```python
from build123d import *

# Parameters (mm, degrees)
BOSS_EXTRUDE1_DEPTH = 6.25
SKETCH2_R           = 2
CUT_EXTRUDE1_DEPTH  = 6.35


with BuildPart() as part:
    # Sketch1 → Boss-Extrude1 (new body)
    with BuildSketch(Plane(origin=(0, 0, 0), x_dir=(1, 0, 0), z_dir=(0, 1, 0))):
        with BuildLine():
            Line((111.125, 0), (187.325, 0))
            ThreePointArc((187.325, 0), (132.458777786, -132.458777786), (0, -187.325))
            Line((0, -187.325), (0, -111.125))
            ThreePointArc((0, -111.125), (78.577241059, -78.577241059), (111.125, 0))
        make_face()
    extrude(amount=BOSS_EXTRUDE1_DEPTH)

    # Sketch2 → Cut-Extrude1 (cut)
    with BuildSketch(Plane(origin=(0, 6.25, 0), x_dir=(1, 0, 0), z_dir=(0, 1, 0))):
        with Locations(Location((21.777652082, -123.507202325, 0), (0, 0, 270))):
            Circle(SKETCH2_R)
        with Locations(Location((123.507202325, -21.777652082, 0), (0, 0, 270))):
            Circle(SKETCH2_R)
        with Locations(Location((26.739648758, -151.648083867, 0), (0, 0, 270))):
            Circle(SKETCH2_R)
        with Locations(Location((151.648083867, -26.739648758, 0), (0, 0, 270))):
            Circle(SKETCH2_R)
    extrude(amount=-CUT_EXTRUDE1_DEPTH, mode=Mode.SUBTRACT)


solid = part.part
```
Source: CAD feature listing. Evaluate the final solid. Frame: model axes, mm. Give positions to 0.01 mm unless a question says otherwise; leave off trailing zeros. Loops run counter-clockwise (first coordinate to the right, second up) from the corner with the lowest first, then second, coordinate; pieces in that order, holes last. Notation, with made-up numbers: (-21, -32) -> (0, -32) arc R16 cw to (0, -14) -> close; hole circle Ø6 at (87, 70.5). An arc over 180 degrees is marked (long way). Put each result on its own line as item: value. Start each with the question number.
1) Material intervals for probe 1 along Z at (x, y) = (25, 4.25); probe 2 along X at (y, z) = (3, 25.5); probe 3 along X at (y, z) = (2.5, 116.5), sorted ascending.
2) Draft query along Z for faces 1 (the face through (133.9, 3.1, 131)), 2 (the face through (28.43, 3.17, 152.72)), 3 (the face through (95, 6.25, 92)). Return one class per face: released by +Z, released by -Z, zero draft, split by the parting line, or undercut.
3) Contact query for flat-ended pins moving along their axis: P1, Ø1.5, axis at y = 2, z = 119.5, coming from the +X side; P2, Ø3, axis at x = 38.5, y = 5, coming from the -Z side; P3, Ø1, axis at x = 90.5, y = 2, coming from the +Z side. Output: stop coordinate, or through.
4) Cut plane C-C (x = 99.5). Return loops of the section in (y, z), then the cut area to 3 significant figures.
5) Cut plane B-B (z = 146). Return loops of the section in (x, y).
6) Cut plane A-A (y = 2). Return loops of the section in (x, z) (3 decimals), then the cut area to 3 significant figures.
Results are:
1. probe 1: z = 108.28 to 150.66, 152.63 to 185.65
1. probe 2: x = 108.16 to 150.08, 153.22 to 185.58
1. probe 3: x = 0 to 146.69
2. face 1: released by +Z
2. face 2: undercut
2. face 3: zero draft
3. P1: stops at x = 144.88
3. P2: stops at z = 103.68
3. P3: stops at z = 164.29
4. outline: (0, 49.48) -> (6.25, 49.48) -> (6.25, 158.71) -> (0, 158.71) -> close
4. area: 683 mm2
5. outline: (0, 0) -> (117.37, 0) -> (117.37, 6.25) -> (0, 6.25) -> close
6. outline: (0, 111.125) arc R111.125 cw to (111.125, 0) -> (187.325, 0) arc R187.325 ccw to (0, 187.325) -> close; hole circle Ø4 at (21.778, 123.507); hole circle Ø4 at (26.74, 151.648); hole circle Ø4 at (123.507, 21.778); hole circle Ø4 at (151.648, 26.74)
6. area: 17,800 mm2
